Build history of the part. All positions in model axes, mm. A direction names the side the tool comes from. Round coordinates to 2 decimals unless told otherwise and drop trailing zeros. Write each loop counter-clockwise with the first axis right and the second up, starting at its lowest first coordinate (ties: lowest second). Pieces come first, ordered by that corner, then holes. Notation, with made-up numbers: (87, 4.5) -> (125, 4.5) arc R19 cw to (125, 16.5) -> close; hole circle Ø5 at (-26, 2). An arc over 180 degrees is marked (long way). Answer in a Markdown table with one row per item. Add a question column.
from build123d import *

# Parameters (mm, degrees)
BOSS_EXTRUDE1_DEPTH = 19.05
CUT_EXTRUDE1_DEPTH  = 12.7
FILLET1_R           = 2.54
CUT_EXTRUDE2_DEPTH  = 12.7


with BuildPart() as part:
    # Sketch1 → Boss-Extrude1 (new body)
    with BuildSketch(Plane(origin=(0, 0, 0), x_dir=(1, 0, 0), z_dir=(0, 1, 0))):
        with BuildLine():
            Line((57.234735331, 57.711554056), (68.22559355, 65.553540024))
            ThreePointArc((68.22559355, 65.553540024), (0, 94.615), (-68.22559355, 65.553540024))
            Line((-68.22559355, 65.553540024), (-57.234735331, 57.711554056))
            ThreePointArc((-57.234735331, 57.711554056), (0, 81.28), (57.234735331, 57.711554056))
        make_face()
    extrude(amount=BOSS_EXTRUDE1_DEPTH)

    # Sketch3 → Cut-Extrude1 (cut)
    with BuildSketch(Plane.XZ):
        with BuildLine():
            Line((-60.379405736, -59.955278859), (-64.043453365, -62.569579718))
            ThreePointArc((-64.043453365, -62.569579718), (0, -89.535), (64.043453365, -62.569579718))
            Line((64.043453365, -62.569579718), (60.379405736, -59.955278859))
            ThreePointArc((60.379405736, -59.955278859), (0, -85.09), (-60.379405736, -59.955278859))
        make_face()
    extrude(amount=-CUT_EXTRUDE1_DEPTH, mode=Mode.SUBTRACT)

    # Fillet1
    fillet1_edges = [part.edges().sort_by_distance(p)[0] for p in [
        (0, 19.05, -81.28),
        (0, 19.05, -94.615),
    ]]
    fillet(fillet1_edges, radius=FILLET1_R)

    # Sketch5 → Cut-Extrude2 (cut)
    with BuildSketch(Plane(origin=(0, 0, 0), x_dir=(-1, 0, 0), z_dir=(0, 1, 0))):
        with BuildLine():
            ThreePointArc((-49.614735331, -61.142175608), (0, -78.74), (49.614735331, -61.142175608))
            Line((49.614735331, -61.142175608), (58.988817486, -74.785572884))
            ThreePointArc((58.988817486, -74.785572884), (0, -95.25), (-58.988817486, -74.785572884))
            Line((-58.988817486, -74.785572884), (-49.614735331, -61.142175608))
        make_face()
    extrude(amount=CUT_EXTRUDE2_DEPTH, mode=Mode.SUBTRACT)


solid = part.part
(1) Saw through at B-B (x = 0). List the corners of the cut face in (y, z) (3 decimals), plus the area to 3 significant figures.
(2) Probe line 1 along X through (y, z) = (8.5, -64); line 2 along X through (y, z) = (3.5, -63); line 3 along X through (y, z) = (9.25, -59). List the from-to ranges inside material, lowest first.
(3) Drop flat-ended pins along their axis: P1, Ø12, axis at x = 40.5, z = -90, coming from the +Y side; P2, Ø2, axis at x = -33, y = 14.5, coming from the -Z side; P3, Ø10, axis at y = 17, z = -72.5, coming from the -X side; P4, Ø1.5, axis at x = 47.5, y = 11, coming from the +Z side. Give the stop position or say it passes through.
(4) Mould opens along Z. For faces 4 (the face through (-60.069, 6.261, -66.394)), 5 (the face through (56, 0, -62)), 6 (the face through (-52.12, 6.26, -64.79)) say: pulls with the +Z half, pulls with the -Z half, needs draft (parallel to the pull), parting line crosses it, or undercut.
(5) Saw through at A-A (y = 3.5). List the corners of the cut face in (x, z) (3 decimals).
(6) Which spindle directions (+Z, -Z, +X, -X, +Y, -Y) get a long thin tool onto all of the face, cutting with end or side? Do faces 1 (the face through (1.07, 13.64, -94.61)), 2 (the face through (-57.167, 6.261, -72.133)), 3 (the face through (56.94, 6.26, -63.23)). Say none if no direction does.
Answer sheet:
| question | item | result |
|---|---|---|
| 1 | outline | (12.7, -94.615) -> (16.51, -94.615) arc R2.54 ccw to (19.05, -92.075) -> (19.05, -83.82) arc R2.54 ccw to (16.51, -81.28) -> (12.7, -81.28) -> close |
| 1 | area | 81.9 mm² |
| 2 | line 1 | x = -66.05 to -62.61, -56.07 to -51.58, 51.58 to 56.07, 62.61 to 66.05 |
| 2 | line 2 | x = -64.65 to -63.62, -57.2 to -51.36, 51.36 to 57.2, 63.62 to 64.65 |
| 2 | line 3 | x = -59.04 to -55.91, 55.91 to 59.04 |
| 3 | P1 | stops at y = 18.97 |
| 3 | P2 | stops at z = -89.04 |
| 3 | P3 | stops at x = -66.28 |
| 3 | P4 | passes through |
| 4 | face 4 | undercut |
| 4 | face 5 | needs draft |
| 4 | face 6 | pulls with the -Z half |
| 5 | outline | (-68.226, -65.554) arc R94.615 ccw to (-58.628, -74.261) -> (-55.745, -70.064) arc R89.535 cw to (-64.043, -62.57) -> close; (-60.379, -59.955) arc R85.09 ccw to (-53.221, -66.391) -> (-51.058, -63.242) arc R81.28 cw to (-57.235, -57.712) -> close; (51.058, -63.242) -> (53.221, -66.391) arc R85.09 ccw to (60.379, -59.955) -> (57.235, -57.712) arc R81.28 cw to start; (55.745, -70.064) -> (58.628, -74.261) arc R94.615 ccw to (68.226, -65.554) -> (64.043, -62.57) arc R89.535 cw to start |
| 6 | face 1 | -Z, +Y, -Y |
| 6 | face 2 | -Z, -Y |
| 6 | face 3 | -Y |
